Geometry check sheet. Reference: the model listing, model coordinates, mm. Face numbers are marked on the shaded views. Give positions to 0.01 mm unless a question says otherwise; leave off trailing zeros. Loops run counter-clockwise (first coordinate to the right, second up) from the corner with the lowest first, then second, coordinate; pieces in that order, holes last.
1. Cross-section at D-D, the plane y = -25.5. State how many separate pieces and enclosed holes the cut face has, plus the area to 3 significant figures.
2. Cross-section at A-A, the plane z = -4.05. Record the cut outline in (x, y), plus the area to 3 significant figures.
3. Cross-section at B-B, the plane x = 77. Record the cut outline in (y, z).
4. Go/stop test with flat-tipped pins: pin 1 Ø2.5 at (y, z) = (-29.5, -3.5) entering from -X; pin 2 Ø1 at (x, y) = (123.5, -58) entering from -Z; pin 3 Ø1 at (y, z) = (-42, -1.5) entering from -X; pin 4 Ø1.5 at (y, z) = (-17, -4) entering from -X. Record where each tip stops, or that it passes through.
5. Cross-section at C-C, the plane y = -40. Record the cut outline in (x, z), plus the area to 3 significant figures.
6. Release check for a two-part mould opening along X. For the marked faces 1 and 2 record: +X half, -X half, draft (parallel to the pull), parting line (faces both ways), or undercut.
7. Material ranges on L1, parallel to X at y = -18.5, z = -2.85; L2, parallel to X at y = -20, z = -1.25; L3, parallel to Z at x = 80, y = -4, recorded low to high.
from build123d import *

# Parameters (mm, degrees)
SKETCH2_W           = 168.310893
SKETCH2_H           = 71
BOSS_EXTRUDE3_DEPTH = 0.7
BOSS_EXTRUDE5_DEPTH = 5


with BuildPart() as part:
    # Sketch2 → Boss-Extrude3 (new body)
    with BuildSketch(Plane.XY):
        with Locations((84.1554465, -35.5)):
            Rectangle(SKETCH2_W, SKETCH2_H)
        Polygon((39.254849, -34.4), (39.254849, -23.4), (32.004849, -6), (32.004849, -17), align=None, mode=Mode.SUBTRACT)
        Polygon((52.004849, -17), (44.754849, -34.4), (44.754849, -23.4), (52.004849, -6), align=None, mode=Mode.SUBTRACT)
        Polygon((37.004849, -6), (42.004849, -18), (47.004849, -6), align=None, mode=Mode.SUBTRACT)
        Polygon((93.004849, -6), (103.004849, -6), (98.004849, -18), align=None, mode=Mode.SUBTRACT)
        Polygon((72.754849, -34.4), (72.754849, -23.4), (80.004849, -6), (80.004849, -17), align=None, mode=Mode.SUBTRACT)
        Polygon((70.004849, -18), (75.004849, -6), (65.004849, -6), align=None, mode=Mode.SUBTRACT)
        Polygon((95.254849, -34.4), (95.254849, -23.4), (88.004849, -6), (88.004849, -17), align=None, mode=Mode.SUBTRACT)
        Polygon((108.004849, -6), (108.004849, -17), (100.754849, -34.4), (100.754849, -23.4), align=None, mode=Mode.SUBTRACT)
        Polygon((60.004849, -17), (67.254849, -34.4), (67.254849, -23.4), (60.004849, -6), align=None, mode=Mode.SUBTRACT)
        Polygon((116.004849, -17), (123.254849, -34.4), (123.254849, -23.4), (116.004849, -6), align=None, mode=Mode.SUBTRACT)
        Polygon((136.004849, -17), (128.754849, -34.4), (128.754849, -23.4), (136.004849, -6), align=None, mode=Mode.SUBTRACT)
        Polygon((126.004849, -18), (131.004849, -6), (121.004849, -6), align=None, mode=Mode.SUBTRACT)
    extrude(amount=BOSS_EXTRUDE3_DEPTH)

    # Sketch2_6 → Boss-Extrude5 (add)
    with BuildSketch(Plane.XY):
        Polygon((9.259849, -6.17), (18.749849, -6.17), (14.004849, -17.558), align=None)
        Polygon((11.084849, -33.55), (11.084849, -23.434), (4.174849, -6.85), (4.174849, -16.966), align=None)
        Polygon((16.924849, -23.434), (23.834849, -6.85), (23.834849, -16.966), (16.924849, -33.55), align=None)
        Polygon((149.259849, -6.17), (158.749849, -6.17), (154.004849, -17.558), align=None)
        Polygon((144.174849, -6.85), (144.174849, -16.966), (151.084849, -33.55), (151.084849, -23.434), align=None)
        Polygon((156.924849, -33.55), (156.924849, -23.434), (163.834849, -6.85), (163.834849, -16.966), align=None)
    extrude(amount=-BOSS_EXTRUDE5_DEPTH)


solid = part.part
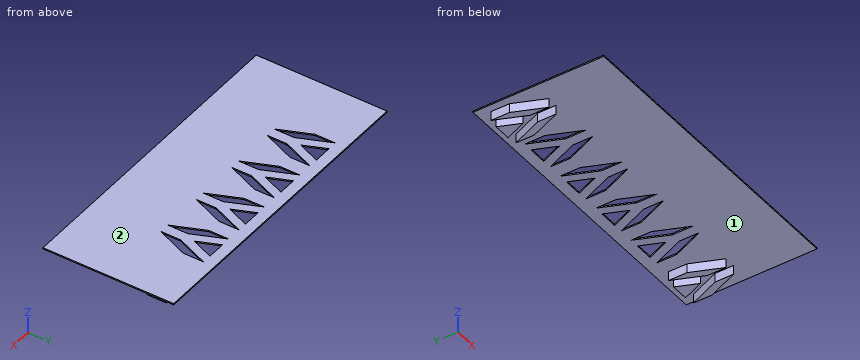
Result:
1. separate pieces: 9
1. enclosed holes: 0
1. area: 164 mm2
2. outline: (4.17, -16.97) - (11.08, -33.55) - (11.08, -23.43) - (4.17, -6.85) - close; (9.26, -6.17) - (14, -17.56) - (18.75, -6.17) - close; (16.92, -33.55) - (23.83, -16.97) - (23.83, -6.85) - (16.92, -23.43) - close; (144.17, -16.97) - (151.08, -33.55) - (151.08, -23.43) - (144.17, -6.85) - close; (149.26, -6.17) - (154, -17.56) - (158.75, -6.17) - close; (156.92, -33.55) - (163.83, -16.97) - (163.83, -6.85) - (156.92, -23.43) - close
2. area: 388 mm2
3. outline: (-71, 0) - (-24.21, 0) - (-24.21, 0.7) - (-71, 0.7) - close; (-13.21, 0) - (0, 0) - (0, 0.7) - (-13.21, 0.7) - close
4. pin 1: stops at x = 8.88
4. pin 2: stops at z = 0
4. pin 3: passes through
4. pin 4: stops at x = 4.17
5. outline: (0, 0) - (168.31, 0) - (168.31, 0.7) - (0, 0.7) - close
5. area: 118 mm2
6. face 1: undercut
6. face 2: draft
7. L1: x = 4.81 to 9.03, 18.98 to 23.2, 144.81 to 149.03, 158.98 to 163.2
7. L2: x = 5.44 to 9.65, 18.36 to 22.57, 145.44 to 149.65, 158.36 to 162.57
7. L3: z = 0 to 0.7
